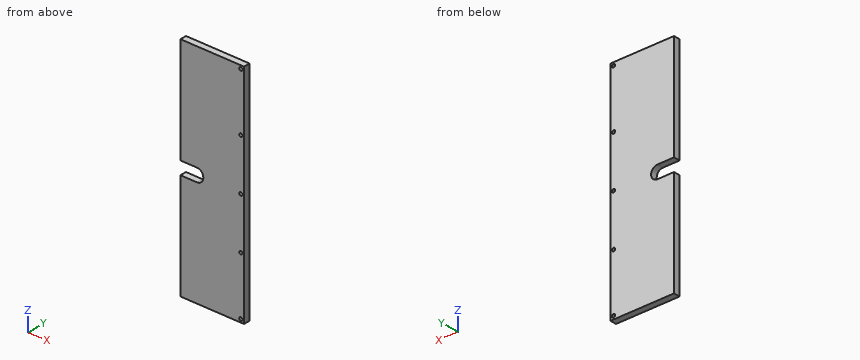
Autodesk Inventor part; units mm, degrees
ref_plane "YZ Plane" through (0, 0, 0) normal (1, 0, 0) x (0, 1, 0)
ref_plane "XZ Plane" through (0, 0, 0) normal (0, 1, 0) x (-1, 0, 0)
ref_plane "XY Plane" through (0, 0, 0) normal (0, 0, 1) x (1, 0, 0)
sketch "Sketch1" plane through (0, 0, 0) normal (0, 1, 0) x (-1, 0, 0)
  line L0 (-50, 175) -> (50, 175)
  line L1 (50, 175) -> (50, -175)
  line L2 (50, -175) -> (-50, -175)
  line L3 (-50, -175) -> (-50, 175)
  line L4 (-50, 175) -> (50, -175) construction
  line L5 (50, 175) -> (-50, -175) construction
  point P0 (0, 0)
  dimension "d0" = 350
  dimension "d1" = 100
extrude "Extrusion1" add sketch "Sketch1" along normal blind 10
sketch "Sketch2" plane through (0, 0, 0) normal (0, -1, 0) x (1, 0, 0)
  circle A0 centre (-24, 0) radius 5
  circle A1 centre (-24, 0) radius 10
  line L0 (-24, 10) -> (-24, -10)
  line L1 (-24, -10) -> (-50, -10)
  line L2 (-50, -10) -> (-50, 10)
  line L3 (-50, 10) -> (-24, 10)
  line L4 (-50, 175) -> (-50, -175)
  point P0 (0, 0)
  dimension "d4" = 20
extrude "Extrusion2" cut sketch "Sketch2" against normal blind 10
sketch "Sketch3" plane through (0, 0, 0) normal (0, -1, 0) x (1, 0, 0)
  line L0 (50, 175) -> (50, -175)
  line L1 (45, 150) -> (45, -150)
  line L2 (0, 0) -> (31.7101, 0) construction
  line L3 (-50, 175) -> (50, 175)
  point P0 (45, 0)
  point P1 (45, 170)
  point P2 (45, 80)
  point P3 (45, -80)
  point P4 (45, -170)
  dimension "d7" = 5
  dimension "d8" = 5
  dimension "d9" = 80
hole "Hole1" at (45, 0, 0) at (45, 0, 170) at (45, 0, 80) at (45, 0, -80) at (45, 0, -170) direction (0, 1, 0) diameter 5 end through all
properties part number "08_Tam_canh_hong"
The listing builds one solid part. Answer for the finished solid, in the listing's coordinates (mm). Round coordinates to 2 decimals unless told otherwise and drop trailing zeros. Loops run counter-clockwise (first coordinate to the right, second up) from the corner with the lowest first, then second, coordinate; pieces in that order, holes last.
1) A cutting plane is placed at A-A on x = -30. Determine the outline of the cut face in (y, z).
Outcome:
outline: (0, -175) - (10, -175) - (10, -10) - (0, -10) - close; (0, 10) - (10, 10) - (10, 175) - (0, 175) - close
2) A cutting plane is placed at B-B on y = 7. Determine the outline of the cut face in (x, z), plus the area to 3 significant figures.
Outcome:
outline: (-50, -175) - (50, -175) - (50, 175) - (-50, 175) - (-50, 10) - (-24, 10) arc R10 cw to (-24, -10) - (-50, -10) - close; hole circle Ø5 at (45, -170); hole circle Ø5 at (45, -80); hole circle Ø5 at (45, 0); hole circle Ø5 at (45, 80); hole circle Ø5 at (45, 170)
area: 34,200 mm2
3) Consider line 1 (Z direction, x = 45, y = 5.5); line 2 (X direction, y = 6, z = 0); line 3 (Z direction, x = -28.5, y = 3.75). Determine where each line is inside the solid, lowest interval first.
Outcome:
line 1: z = -175 to -172.5, -167.5 to -82.5, -77.5 to -2.5, 2.5 to 77.5, 82.5 to 167.5, 172.5 to 175
line 2: x = -14 to 42.5, 47.5 to 50
line 3: z = -175 to -10, 10 to 175
